Here's the drawing with two shaded views (mm, measured from the low corner). I have some questions. A direction names the side the tool comes from. Give positions to 0.01 mm unless a question says otherwise; leave off trailing zeros. Loops run counter-clockwise (first coordinate to the right, second up) from the corner with the lowest first, then second, coordinate; pieces in that order, holes last.
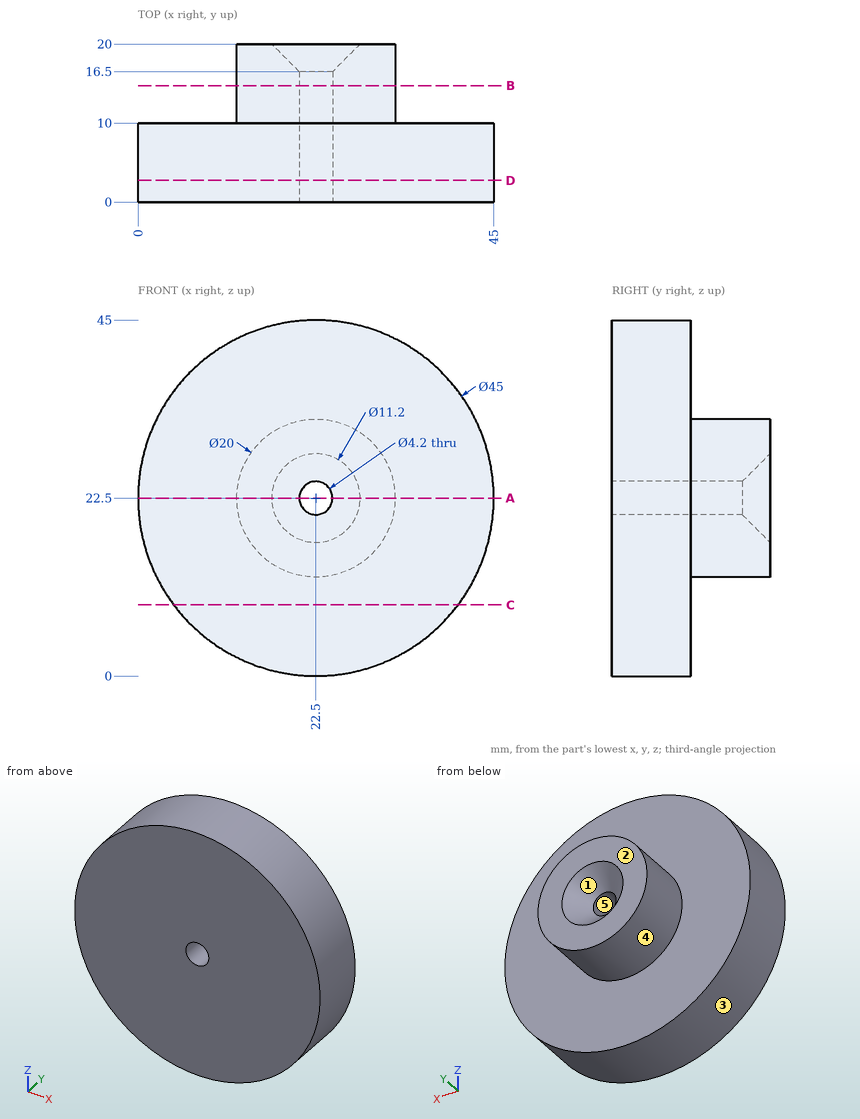
(1) Thinking about a two-plate mould opening in Z: for the marked faces 1, 2 and 3, which applies, pulls with the +Z half, pulls with the -Z half, needs draft (parallel to the pull), parting line crosses it, or undercut?
Returned:
face 1: undercut
face 2: needs draft
face 3: parting line crosses it
(2) Suppose I cut it at D-D on y = 2.75. List the corners of the cut face in (x, z) for me.
Returned:
outline: circle Ø45 at (22.5, 22.5); hole circle Ø4.2 at (22.5, 22.5)
(3) Suppose I cut it at C-C on z = 9. List the corners of the cut face in (x, y) for me, plus the area to 3 significant figures.
Returned:
outline: (4.5, 0) - (40.5, 0) - (40.5, 10) - (4.5, 10) - close
area: 360 mm2
(4) Suppose I cut it at A-A on z = 22.5. List the corners of the cut face in (x, y) for me, plus the area to 3 significant figures.
Returned:
outline: (0, 0) - (20.4, 0) - (20.4, 16.5) - (16.9, 20) - (12.5, 20) - (12.5, 10) - (0, 10) - close; (24.6, 0) - (45, 0) - (45, 10) - (32.5, 10) - (32.5, 20) - (28.1, 20) - (24.6, 16.5) - close
area: 554 mm2
(5) Will these pins go through, and if not, where does the flat tip stop? P1, Ø10, axis at x = 30.5, y = 6, coming from the -Z side; P2, Ø12, axis at y = 2.5, z = 23, coming from the +X side; P3, Ø6, axis at y = 14.5, z = 33, coming from the +X side; P4, Ø5, axis at x = 39.5, z = 34, coming from the +Y side.
Returned:
P1: stops at z = 0.2
P2: stops at x = 45
P3: stops at x = 29.11
P4: stops at y = 10
(6) Which directions (+Z, -Z, +X, -X, +Y, -Y) give clear straight access to the entire face, cutting with the end or side of a thin tool? Please do the marked faces 4 and 5.
Returned:
face 4: +Y
face 5: +Y, -Y
(7) Suppose I cut it at B-B on y = 14.75. List the corners of the cut face in (x, z) for me, plus the area to 3 significant figures.
Returned:
outline: circle Ø20 at (22.5, 22.5); hole circle Ø4.2 at (22.5, 22.5)
area: 300 mm2
(8) Please list where these lines run through material, in increasing order: probe 1 along Z at (x, y) = (22.5, 5); probe 2 along Y at (x, z) = (27, 6.5); probe 3 along Z at (x, y) = (22, 9.75).
Returned:
probe 1: z = 0 to 20.4, 24.6 to 45
probe 2: y = 0 to 10
probe 3: z = 0.01 to 20.46, 24.54 to 44.99
